```python
from build123d import *

# Parameters (mm, degrees)
F3_DEPTH  = 240
F5_DEPTH  = 20
F6_W      = 112
F6_H      = 241.106075
F7_DEPTH  = 25
F8_W      = 70.001994
F8_H      = 85
F9_DEPTH  = 25
F10_W     = 50
F10_H     = 198.001994
F11_DEPTH = 50


with BuildPart() as f3:
    # F2 (on face) → F3 (new body)
    with BuildSketch(Plane.XY):
        Polygon((-627, -343.001994), (-627, -273), (-627, -187), (-765, -187), (-877, -187), (-925, -187), (-925, -427.001994), (-627, -427.001994), align=None)
        Polygon((-765, -208), (-648, -208), (-648, -273), (-648, -343.001994), (-648, -406.001994), (-904, -406.001994), (-904, -208), (-877, -208), align=None, mode=Mode.SUBTRACT)
    extrude(amount=F3_DEPTH)

    # F4 (on face) → F5 (join)
    with BuildSketch(Plane.XY):
        Polygon((-648, -273), (-648, -208), (-765, -208), (-877, -208), (-904, -208), (-904, -406.001994), (-648, -406.001994), (-648, -343.001994), align=None)
    extrude(amount=F5_DEPTH)

    # F6 (on face) → F7 (cut)
    with BuildSketch(Plane(origin=(0, -187, 0), x_dir=(-1, 0, 0), z_dir=(0, 1, 0))):
        with Locations((821, 140.553037)):
            Rectangle(F6_W, F6_H)
    extrude(amount=-F7_DEPTH, mode=Mode.SUBTRACT)

    # F8 (on face) → F9 (cut)
    with BuildSketch(Plane.YZ.offset(-627)):
        with Locations((-308.000997, 177.5)):
            Rectangle(F8_W, F8_H)
    extrude(amount=-F9_DEPTH, mode=Mode.SUBTRACT)

    # F10 (on face) → F11 (join)
    with BuildSketch(Plane.XY.offset(20)):
        with Locations((-673, -307.000997)):
            Rectangle(F10_W, F10_H)
    extrude(amount=F11_DEPTH)


solid = f3.part
```
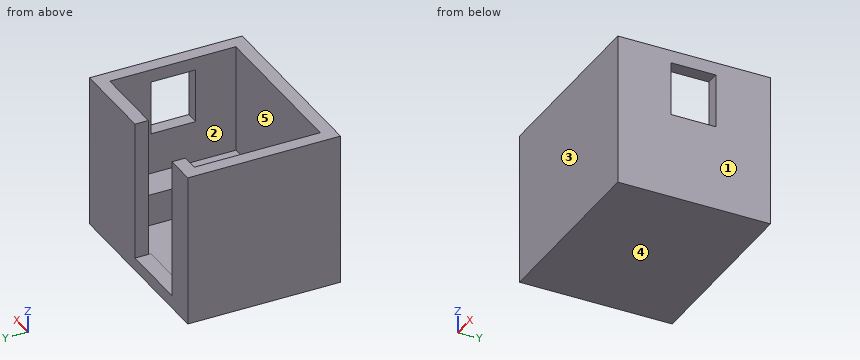
Input: part model. Units: mm. Frame: model coordinates. Face numbers are marked on the shaded views. A direction names the side the tool comes from. Coordinates: 2 decimals unless noted, no trailing zeros. Order: outer loops, then holes, each group sorted by start corner. A loop starts at its lowest first (then second) coordinate and runs counter-clockwise, first axis right, second up. Notation, with made-up numbers: (-10, 26) - (1, 26) arc R10 ccw to (1, 38) - close; hole circle Ø3 at (-21, 56.25). An arc over 180 degrees is marked (long way). Return JSON: item names as keys, results as strings.
Q1. Cut plane D-D (z = 127). Return loops of the section in (x, y).
The answers:
{"outline": "(-925, -427) - (-627, -427) - (-627, -187) - (-765, -187) - (-765, -208) - (-648, -208) - (-648, -406) - (-904, -406) - (-904, -208) - (-877, -208) - (-877, -187) - (-925, -187) - close"}
Q2. First-contact query: pin 1 (12.5 mm diameter, centred on x = -845.5, y = -194, fed in from +Z); pin 2 (1 mm diameter, centred on x = -809, z = 153.5, fed in from +Y); pin 3 (2 mm diameter, centred on x = -867.5, y = -323, fed in from -Z); pin 4 (15 mm diameter, centred on x = -662.5, y = -306, fed in from +Z). Flat tips, straight axial feed; report the tip coordinate or a pass-through.
The answers:
{"pin 1": "stops at z = 20", "pin 2": "stops at y = -406", "pin 3": "stops at z = 0", "pin 4": "stops at z = 70"}
Q3. Cut plane A-A (y = -332.5). Return loops of the section in (x, z).
The answers:
{"outline": "(-925, 0) - (-627, 0) - (-627, 135) - (-648, 135) - (-648, 70) - (-698, 70) - (-698, 20) - (-904, 20) - (-904, 240) - (-925, 240) - close; (-648, 220) - (-627, 220) - (-627, 240) - (-648, 240) - close"}
Q4. Access query for the marked faces 1 and 2. Directions: +Z, -Z, +X, -X, +Y, -Y. A direction counts if a zero-diameter tool reaches every point of the face in a straight line with its end or side. Return the directions, or none.
The answers:
{"face 1": "+Z, -Z, +X, +Y, -Y", "face 2": "+Z"}
Q5. Ray query, probe 1 along X at (y, z) = (-300, 119.5); probe 2 along Y at (x, z) = (-748, 52); probe 3 along X at (y, z) = (-392.5, 28.5). Return the intervals inside material, ascending.
The answers:
{"probe 1": "x = -925 to -904, -648 to -627", "probe 2": "y = -427 to -406, -208 to -187", "probe 3": "x = -925 to -904, -698 to -627"}
Q6. Cut plane B-B (z = 206). Return loops of the section in (x, y).
The answers:
{"outline": "(-925, -427) - (-627, -427) - (-627, -343) - (-648, -343) - (-648, -406) - (-904, -406) - (-904, -208) - (-877, -208) - (-877, -187) - (-925, -187) - close; (-765, -208) - (-648, -208) - (-648, -273) - (-627, -273) - (-627, -187) - (-765, -187) - close"}
Q7. Draft query along Y for the marked faces 3, 4 and 5. Return one class per face: +Y half, -Y half, draft (parallel to the pull), parting line (faces both ways), or undercut.
The answers:
{"face 3": "-Y half", "face 4": "draft", "face 5": "undercut"}
Q8. Cut plane C-C (x = -690.5). Return loops of the section in (y, z), then the cut area to 3 significant figures.
The answers:
{"outline": "(-427, 0) - (-187, 0) - (-187, 240) - (-208, 240) - (-208, 70) - (-406, 70) - (-406, 240) - (-427, 240) - close", "area": "23,900 mm2"}
